Source: three-view drawing plus pictorial views. Frame: mm from the lowest corner of the part. Give positions to 0.01 mm unless a question says otherwise; leave off trailing zeros. Write each loop counter-clockwise with the first axis right and the second up, starting at its lowest first coordinate (ties: lowest second). Pieces come first, ordered by that corner, then holes. Notation, with made-up numbers: (27, -24.75) -> (75, -24.75) arc R15 cw to (75, -20.75) -> close; hole circle Ø6 at (44, 16). An arc over 180 degrees is marked (long way). Answer in a Markdown table with one row per item. Add a question column.
Item 1: Section query A-A on x = 10. Output: boundary loops of the cut face in (y, z), plus the area to 3 significant figures.
Item 2: Section query C-C on y = 1.1. Output: boundary loops of the cut face in (x, z), plus the area to 3 significant figures.
Item 3: Material intervals for probe 1 along Z at (x, y) = (10, 1.05); probe 2 along X at (y, z) = (0.35, 5.5); probe 3 along Z at (x, y) = (18.5, 0.7), sorted ascending. Write a range as from..to.
Item 4: Section query B-B on z = 5.5. Output: boundary loops of the cut face in (x, y), plus the area to 3 significant figures.
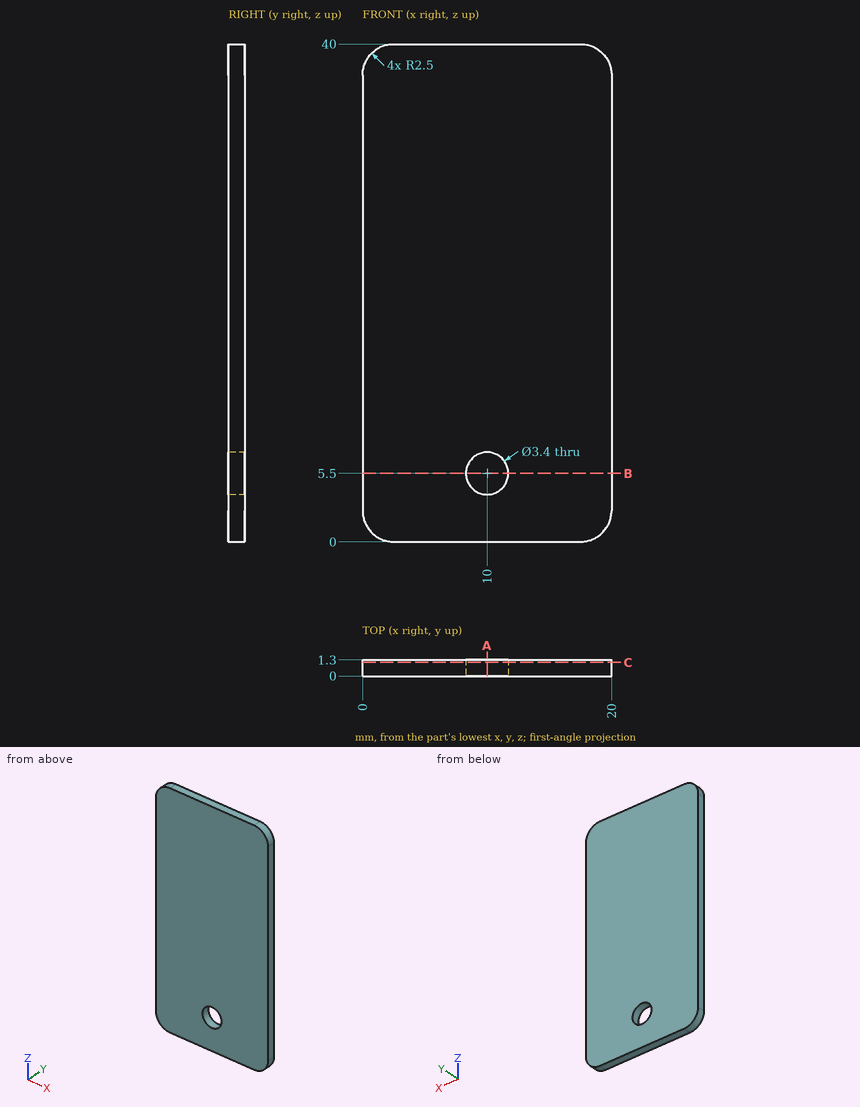
Findings below:
| question | item | result |
|---|---|---|
| 1 | outline | (0, 0) -> (1.3, 0) -> (1.3, 3.8) -> (0, 3.8) -> close; (0, 7.2) -> (1.3, 7.2) -> (1.3, 40) -> (0, 40) -> close |
| 1 | area | 47.6 mm^2 |
| 2 | outline | (0, 2.5) arc R2.5 ccw to (2.5, 0) -> (17.5, 0) arc R2.5 ccw to (20, 2.5) -> (20, 37.5) arc R2.5 ccw to (17.5, 40) -> (2.5, 40) arc R2.5 ccw to (0, 37.5) -> close; hole circle Ø3.4 at (10, 5.5) |
| 2 | area | 786 mm^2 |
| 3 | probe 1 | z = 0..3.8, 7.2..40 |
| 3 | probe 2 | x = 0..8.3, 11.7..20 |
| 3 | probe 3 | z = 0.21..39.79 |
| 4 | outline | (0, 0) -> (8.3, 0) -> (8.3, 1.3) -> (0, 1.3) -> close; (11.7, 0) -> (20, 0) -> (20, 1.3) -> (11.7, 1.3) -> close |
| 4 | area | 21.6 mm^2 |
